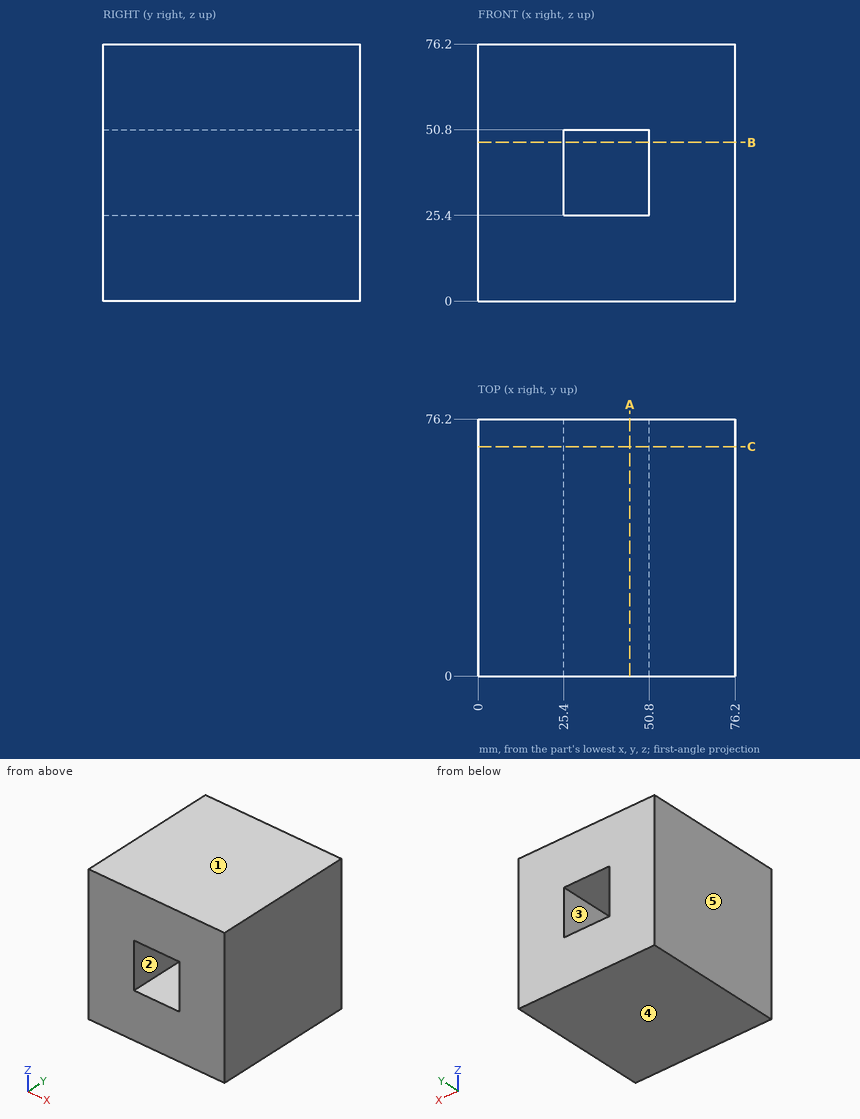
Answer from the drawing. Dimensions are ordinates in mm from the lowest x, y and z of the part. A direction names the side the tool comes from. Round coordinates to 2 decimals unless told otherwise and drop trailing zeros. Loops run counter-clockwise (first coordinate to the right, second up) from the corner with the lowest first, then second, coordinate; pieces in that order, holes last. Notation, with made-up numbers: (34.5, 66.25) - (78.5, 66.25) arc R15 ccw to (78.5, 85.25) - close; hole circle Ø5 at (-29.5, -1). An arc over 180 degrees is marked (long way). Return JSON: item names as keys, results as strings. Group by question number.
1. The mould has two halves that part along X. Classify the marked faces 3, 4 and 5: pulls with the +X half, pulls with the -X half, needs draft (parallel to the pull), parting line crosses it, or undercut.
2. The part is cut by section C-C on y = 68. Determine the outline of the cut face in (x, z), then the cut area to 3 significant figures.
3. The part is cut by section B-B on z = 47. Determine the outline of the cut face in (x, y), then the cut area to 3 significant figures.
4. Which of the six approach directions +Z, -Z, +X, -X, +Y, -Y give full straight-line access (tool end or side, diameter ignored) to the marked faces 1 and 2?
5. The part is cut by section A-A on x = 45. Determine the outline of the cut face in (y, z), then the cut area to 3 significant figures.
6. Consider probe 1 along X at (y, z) = (47.5, 42). Determine where the line is inside the solid, lowest interval first.
Resolved:
{
 "1": {"face 3": "undercut", "face 4": "needs draft", "face 5": "pulls with the -X half"},
 "2": {"outline": "(0, 0) - (76.2, 0) - (76.2, 76.2) - (0, 76.2) - close; hole (25.4, 25.4) - (50.8, 25.4) - (50.8, 50.8) - (25.4, 50.8) - close", "area": "5,160 mm²"},
 "3": {"outline": "(0, 0) - (25.4, 0) - (25.4, 76.2) - (0, 76.2) - close; (50.8, 0) - (76.2, 0) - (76.2, 76.2) - (50.8, 76.2) - close", "area": "3,870 mm²"},
 "4": {"face 1": "+Z, +X, -X, +Y, -Y", "face 2": "+Y, -Y"},
 "5": {"outline": "(0, 0) - (76.2, 0) - (76.2, 25.4) - (0, 25.4) - close; (0, 50.8) - (76.2, 50.8) - (76.2, 76.2) - (0, 76.2) - close", "area": "3,870 mm²"},
 "6": {"probe 1": "x = 0 to 25.4, 50.8 to 76.2"}
}
